Geometry: see drawing. Coordinates: mm, zero at the bounding-box minimum. Round coordinates to 2 decimals unless told otherwise and drop trailing zeros. Order: outer loops, then holes, each group sorted by start corner. A loop starts at its lowest first (then second) coordinate and runs counter-clockwise, first axis right, second up. Notation, with made-up numbers: (26.25, 25.5) - (54.25, 25.5) arc R11 cw to (54.25, 46.5) - close; hole circle Ø7 at (-30.75, 5). An arc over 180 degrees is marked (long way). Put each result on its own line as item: value. Start each with the question number.
1) Contact query for flat-ended pins moving along their axis: P1, Ø1, axis at y = 12, z = 34.5, coming from the -X side; P2, Ø8, axis at x = 69.5, y = 3.5, coming from the -Z side; P3, Ø3, axis at y = 6.5, z = 96.5, coming from the -X side; P4, Ø5, axis at x = 22.5, z = 53.5, coming from the -Y side (3 decimals). Output: stop coordinate, or through.
2) Section C-C on y = 4. Output: boundary loops of the cut face in (x, z), then the cut area to 3 significant figures.
3) Section B-B on z = 70. Output: boundary loops of the cut face in (x, y) (3 decimals), then the cut area to 3 significant figures.
4) Section A-A on y = 16.5. Output: boundary loops of the cut face in (x, z).
5) Line query: probe 1 along X at (y, z) = (11, 88); probe 2 along Y at (x, z) = (51.5, 17) (3 decimals); probe 3 along Z at (x, y) = (93, 9). Output: solid intervals per line, ascending. Write a range as [from, to].
6) Section D-D on x = 91. Output: boundary loops of the cut face in (y, z) (3 decimals), then the cut area to 3 significant figures.
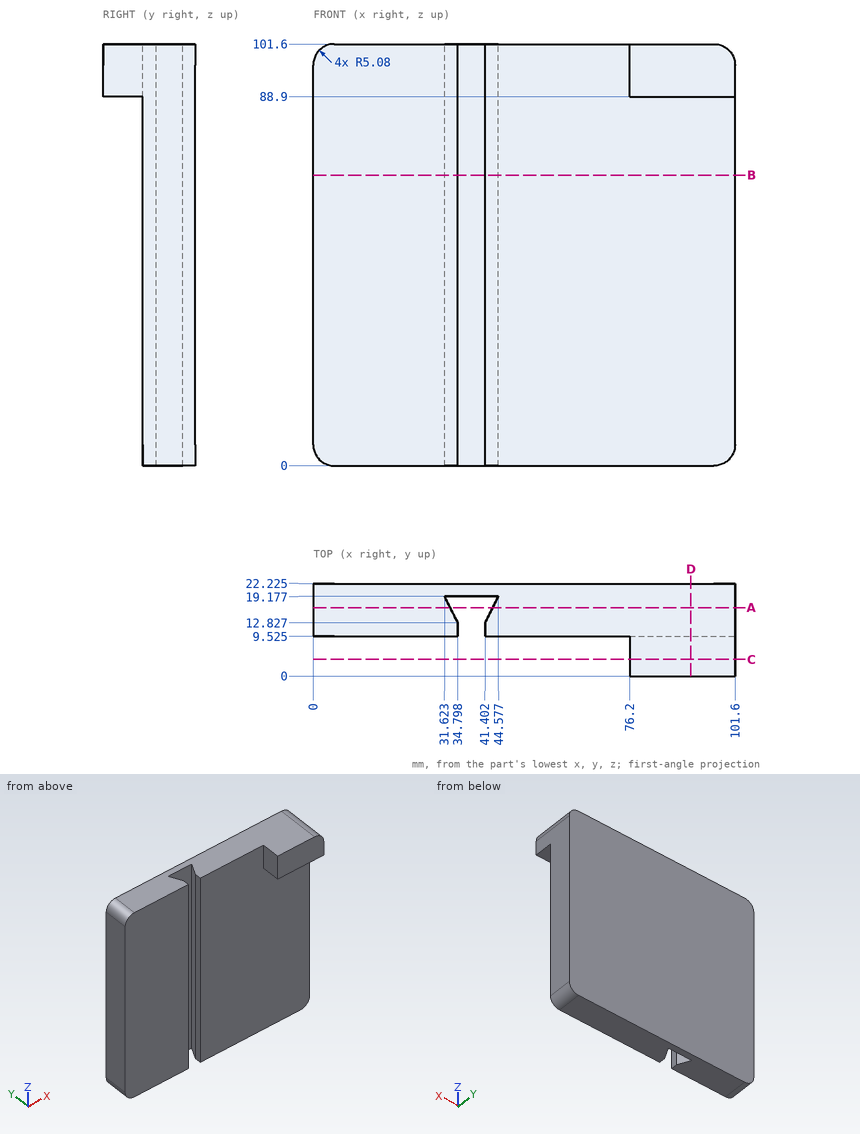
Answer sheet:
1. P1: x = 0
1. P2: through
1. P3: x = 76.2
1. P4: y = 9.525
2. outline: (76.2, 88.9) - (101.6, 88.9) - (101.6, 96.52) arc R5.08 ccw to (96.52, 101.6) - (76.2, 101.6) - close
2. area: 317 mm^2
3. outline: (0, 9.525) - (34.798, 9.525) - (34.798, 12.827) - (31.623, 19.177) - (44.577, 19.177) - (41.402, 12.827) - (41.402, 9.525) - (101.6, 9.525) - (101.6, 22.225) - (0, 22.225) - close
3. area: 1,210 mm^2
4. outline: (0, 5.08) arc R5.08 ccw to (5.08, 0) - (32.96, 0) - (32.96, 101.6) - (5.08, 101.6) arc R5.08 ccw to (0, 96.52) - close; (43.24, 0) - (96.52, 0) arc R5.08 ccw to (101.6, 5.08) - (101.6, 96.52) arc R5.08 ccw to (96.52, 101.6) - (43.24, 101.6) - close
5. probe 1: [0, 34.8], [41.4, 101.6]
5. probe 2: [9.525, 22.225]
5. probe 3: [88.9, 101.6]
6. outline: (0, 88.9) - (9.525, 88.9) - (9.525, 0) - (22.225, 0) - (22.225, 101.6) - (0, 101.6) - close
6. area: 1,410 mm^2
